from build123d import *

# Parameters (mm, degrees)
IZIM1_R                     = 20
Y_KSEKLIK_EKSTR_ZYON1_DEPTH = 35
IZIM1_4_R                   = 20
IZIM1_4_R_2                 = 7.5
Y_KSEKLIK_EKSTR_ZYON2_DEPTH = 15
IZIM1_5_R                   = 10
KES_EKSTR_ZYON1_DEPTH       = 35


with BuildPart() as part:
    # izim1 → Y_kseklik-Ekstr_zyon1 (new body)
    with BuildSketch(Plane.XY):
        with Locations((-29.903991686, 4.831419272)):
            Circle(IZIM1_R)
    extrude(amount=Y_KSEKLIK_EKSTR_ZYON1_DEPTH)

    # izim1_4 → Y_kseklik-Ekstr_zyon2 (add)
    with BuildSketch(Plane.XY):
        with BuildLine():
            Line((-59.079607017, 11.815935722), (-49.412372708, 48.640209122))
            ThreePointArc((-49.412372708, 48.640209122), (-44.065545927, 56.70853693), (-34.903991686, 59.831419272))
            Line((-34.903991686, 59.831419272), (7.146594433, 59.831419272))
            Line((7.146594433, 59.831419272), (55.096008314, 59.831419272))
            ThreePointArc((55.096008314, 59.831419272), (70.096008314, 44.831419272), (55.096008314, 29.831419272))
            Line((55.096008314, 29.831419272), (46.085321375, 29.831419272))
            ThreePointArc((46.085321375, 29.831419272), (16.92570157, 20.448122398), (-1.28938346, -4.179917815))
            ThreePointArc((-1.28938346, -4.179917815), (-37.906835858, -24.081458226), (-59.079607017, 11.815935722))
        make_face()
        with Locations((-29.903991686, 4.831419272)):
            Circle(IZIM1_4_R, mode=Mode.SUBTRACT)
        with Locations((-34.903991686, 44.831419272)):
            Circle(IZIM1_4_R_2, mode=Mode.SUBTRACT)
        with BuildLine():
            ThreePointArc((55.096008314, 38.831419272), (61.096008314, 44.831419272), (55.096008314, 50.831419272))
            Line((55.096008314, 50.831419272), (15.096008314, 50.831419272))
            ThreePointArc((15.096008314, 50.831419272), (9.096008314, 44.831419272), (15.096008314, 38.831419272))
            Line((15.096008314, 38.831419272), (55.096008314, 38.831419272))
        make_face(mode=Mode.SUBTRACT)
    extrude(amount=Y_KSEKLIK_EKSTR_ZYON2_DEPTH)

    # izim1_5 → Kes-Ekstr_zyon1 (cut)
    with BuildSketch(Plane.XY):
        with Locations((-29.903991686, 4.831419272)):
            Circle(IZIM1_5_R)
    extrude(amount=KES_EKSTR_ZYON1_DEPTH, mode=Mode.SUBTRACT)


solid = part.part
Build history of the part. All positions in model axes, mm. A direction names the side the tool comes from. Coordinates: 2 decimals unless noted, no trailing zeros. Order: outer loops, then holes, each group sorted by start corner. A loop starts at its lowest first (then second) coordinate and runs counter-clockwise, first axis right, second up. Notation, with made-up numbers: (-39, -33) - (1, -33) arc R23 cw to (1, 0) - close; hole circle Ø9 at (-27, 26.25). An arc over 180 degrees is marked (long way). Write each question's results on one line, items separated by ' | '. Start each with the question number.
Item 1: Flat gauge pins, fed straight in: pin 1 (3 mm diameter, centred on y = 16.5, z = 15.5, fed in from -X); pin 2 (2 mm diameter, centred on y = -13, z = 12, fed in from +X); pin 3 (12 mm diameter, centred on x = 31, z = 6.5, fed in from -Y). Where does each tip first touch, or does it go through?
Item 2: Wall check: probe 1 along Y at (x, z) = (46, 13); probe 2 along Z at (x, y) = (-53, -11); probe 3 along Y at (x, z) = (-26, 11). Give the ranges that are in metal, low to high. Write a range as [from, to].
Item 3: Mould opens along X. For faces 5 (the face through (-8, 27, 0)), 6 (the face through (-44.174, 56.624, 7.395)), 7 (the face through (61.095, 44.699, 7.395)) say: released by +X, released by -X, zero draft, split by the parting line, or undercut.
Item 4: Band-saw the part on C-C on x = -45. Write the cut outline in (y, z), and give its area (3 significant figures).
Item 5: Band-saw the part on B-B on z = 6.5. Write the cut outline in (x, y).
Item 6: Tool access for faces 1 (the face through (-49.885, 5.711, 24.86)), 2 (the face through (51, 29.831, 7)), 3 (the face through (9.1, 45, 7.4)), 4 (the face through (-54.314, 29.97, 7.395)): list every direction of +Z, -Z, +X, -X, +Y, -Y with a clear straight run to the whole face (end or side of a thin tool).
Item 7: Band-saw the part on D-D on x = 29. Write the cut outline in (y, z), and give its area (3 significant figures).
Item 8: Band-saw the part on A-A on x = 49. Write the cut outline in (y, z), and give its area (3 significant figures).
Numbers:
1) pin 1: x = -58.22 | pin 2: x = -5.07 | pin 3: y = 25.17
2) probe 1: [29.83, 38.83], [50.83, 59.83] | probe 2: [0, 15] | probe 3: [-24.91, -4.38], [14.04, 59.83]
3) face 5: zero draft | face 6: released by -X | face 7: undercut
4) outline: (-21.09, 0) - (55.93, 0) - (55.93, 15) - (17.95, 15) - (17.95, 35) - (-8.29, 35) - (-8.29, 15) - (-21.09, 15) - close | area: 1,680 mm^2
5) outline: (-59.08, 11.82) arc R30 ccw to (-1.29, -4.18) arc R50 cw to (46.09, 29.83) - (55.1, 29.83) arc R15 ccw to (55.1, 59.83) - (-34.9, 59.83) arc R15 ccw to (-49.41, 48.64) - close; hole circle Ø15 at (-34.9, 44.83); hole circle Ø20 at (-29.9, 4.83); hole (15.1, 38.83) - (55.1, 38.83) arc R6 ccw to (55.1, 50.83) - (15.1, 50.83) arc R6 ccw to start
6) face 1: +Z | face 2: +Z, -Z, +X, -Y | face 3: +Z, -Z | face 4: +Z, -Z, -X, +Y
7) outline: (26.82, 0) - (38.83, 0) - (38.83, 15) - (26.82, 15) - close; (50.83, 0) - (59.83, 0) - (59.83, 15) - (50.83, 15) - close | area: 315 mm^2
8) outline: (29.83, 0) - (38.83, 0) - (38.83, 15) - (29.83, 15) - close; (50.83, 0) - (59.83, 0) - (59.83, 15) - (50.83, 15) - close | area: 270 mm^2
